from build123d import *

# Parameters (mm, degrees)
F0_R     = 16
F0_R_2   = 3
F1_DEPTH = 10
F2_W     = 20
F2_H     = 5
F3_DEPTH = 25
F5_D     = 4


with BuildPart() as f1:
    # F0 (on Top) → F1 (new body)
    with BuildSketch(Plane.XY):
        Circle(F0_R)
        with Locations((0, -11.75)):
            Circle(F0_R_2, mode=Mode.SUBTRACT)
        with Locations((0, 11.75)):
            Circle(F0_R_2, mode=Mode.SUBTRACT)
    extrude(amount=F1_DEPTH)

    # F2 (on face) → F3 (join)
    with BuildSketch(Plane(origin=(0, 0, 0), x_dir=(1, 0, 0), z_dir=(0, 0, -1))):
        Rectangle(F2_W, F2_H)
    extrude(amount=F3_DEPTH)

    # F5 (through all)
    with Locations(Plane(origin=(0, 2.5, 0), x_dir=(-1, 0, 0), z_dir=(0, 1, 0))):
        with Locations((0, -20)):
            Hole(F5_D / 2)


solid = f1.part
Verification items for the finished model (mm, model axes). A direction names the side the tool comes from. Give positions to 0.01 mm unless a question says otherwise; leave off trailing zeros. Write each loop counter-clockwise with the first axis right and the second up, starting at its lowest first coordinate (ties: lowest second). Pieces come first, ordered by that corner, then holes.
(1) Cross-section at A-A (x = 0). Enter the section's corners in (y, z).
(2) Cross-section at B-B (z = -20). Enter the section's corners in (x, y), plus the area to 3 significant figures.
(3) Mould release check, pull along X, two halves, no side actions. Record for faces 6 (the face through (10, 0, -12)), 7 (the face through (-0.65, 8.82, 4.93)), 8 (the face through (-3.47, -15.62, 4.93)): +X half, -X half, draft (parallel to the pull), parting line (faces both ways), or undercut.
(4) Material ranges on line 1 (Y direction, x = 0, z = 4.5); line 2 (Z direction, x = 0, y = -0.2); line 3 (Y direction, x = 5.5, z = -8.5), recorded low to high.
(5) Cross-section at D-D (z = 6). Enter the section's corners in (x, y).
(6) Access from +Z, -Z, +X, -X, +Y, -Y to the whole of each face (thin tool, end or side, straight path). Record for faces 1 (the face through (0, 2.5, -12)), 2 (the face through (0, -2.5, -12)), 3 (the face through (0, 0, 10)), 4 (the face through (0, 0, -25)), 5 (the face through (-10, 0, -12)).
(7) Gauge pin test, flat ends, axial feed: pin 1 (1.5 mm diameter, centred on y = -0.5, z = -9.5, fed in from +X); pin 2 (12 mm diameter, centred on x = -5.5, z = -9.5, fed in from +Y); pin 3 (3.5 mm diameter, centred on x = 0, y = -11.75, fed in from +Z); pin 4 (2.5 mm diameter, centred on y = 0, z = -10.5, fed in from -X). Record the tip position at first contact, or that the pin passes through.
(8) Cross-section at C-C (y = -13). Enter the section's corners in (x, z), plus the area to 3 significant figures.
Worked out:
1. outline: (-16, 0) - (-14.75, 0) - (-14.75, 10) - (-16, 10) - close; (-8.75, 0) - (-2.5, 0) - (-2.5, -18) - (2.5, -18) - (2.5, 0) - (8.75, 0) - (8.75, 10) - (-8.75, 10) - close; (-2.5, -25) - (2.5, -25) - (2.5, -22) - (-2.5, -22) - close; (14.75, 0) - (16, 0) - (16, 10) - (14.75, 10) - close
2. outline: (-10, -2.5) - (-2, -2.5) - (-2, 2.5) - (-10, 2.5) - close; (2, -2.5) - (10, -2.5) - (10, 2.5) - (2, 2.5) - close
2. area: 80.0 mm2
3. face 6: +X half
3. face 7: undercut
3. face 8: parting line
4. line 1: y = -16 to -14.75, -8.75 to 8.75, 14.75 to 16
4. line 2: z = -25 to -22, -18 to 10
4. line 3: y = -2.5 to 2.5
5. outline: circle Ø32 at (0, 0); hole circle Ø6 at (0, -11.75); hole circle Ø6 at (0, 11.75)
6. face 1: -Z, +X, -X, +Y
6. face 2: -Z, +X, -X, -Y
6. face 3: +Z, +X, -X, +Y, -Y
6. face 4: -Z, +X, -X, +Y, -Y
6. face 5: -Z, -X, +Y, -Y
7. pin 1: stops at x = 10
7. pin 2: stops at y = 2.5
7. pin 3: passes through
7. pin 4: stops at x = -10
8. outline: (-9.33, 0) - (-2.73, 0) - (-2.73, 10) - (-9.33, 10) - close; (2.73, 0) - (9.33, 0) - (9.33, 10) - (2.73, 10) - close
8. area: 132 mm2
